Autodesk Inventor part; units mm, degrees
ref_plane "YZ Plane" through (0, 0, 0) normal (1, 0, 0) x (0, 1, 0)
ref_plane "XZ Plane" through (0, 0, 0) normal (0, 1, 0) x (-1, 0, 0)
ref_plane "XY Plane" through (0, 0, 0) normal (0, 0, 1) x (1, 0, 0)
sketch "스케치1" plane through (0, 0, 0) normal (0, 1, 0) x (-1, 0, 0)
  line L0 (24.9446, -24.9446) -> (9.1304, -34.075)
  line L1 (9.1304, -34.075) -> (-9.1304, -34.075)
  line L2 (-9.1304, -34.075) -> (-24.9446, -24.9446)
  line L3 (-24.9446, -24.9446) -> (-34.075, -9.1304)
  line L4 (-34.075, -9.1304) -> (-34.075, 9.1304)
  line L5 (-34.075, 9.1304) -> (-24.9446, 24.9446)
  line L6 (-24.9446, 24.9446) -> (-9.1304, 34.075)
  line L7 (-9.1304, 34.075) -> (9.1304, 34.075)
  line L8 (9.1304, 34.075) -> (24.9446, 24.9446)
  line L9 (24.9446, 24.9446) -> (34.075, 9.1304)
  line L10 (34.075, 9.1304) -> (34.075, -9.1304)
  line L11 (34.075, -9.1304) -> (24.9446, -24.9446)
  line L12 (9.9878, -37.275) -> (-9.9878, -37.275)
  line L13 (-9.9878, -37.275) -> (-27.2872, -27.2872)
  line L14 (-27.2872, -27.2872) -> (-37.275, -9.9878)
  line L15 (-37.275, -9.9878) -> (-37.275, 9.9878)
  line L16 (-37.275, 9.9878) -> (-27.2872, 27.2872)
  line L17 (-27.2872, 27.2872) -> (-9.9878, 37.275)
  line L18 (-9.9878, 37.275) -> (9.9878, 37.275)
  line L19 (9.9878, 37.275) -> (27.2872, 27.2872)
  line L20 (27.2872, 27.2872) -> (37.275, 9.9878)
  line L21 (37.275, 9.9878) -> (37.275, -9.9878)
  line L22 (37.275, -9.9878) -> (27.2872, -27.2872)
  line L23 (27.2872, -27.2872) -> (9.9878, -37.275)
  point P0 (0, 0)
  point P1 (0, 0)
  point P2 (0, 0)
  dimension "d0" = 70.554
  dimension "d1" = 3.2
extrude "돌출1" add sketch "스케치1" along normal blind 3.7 contours L0 L1 L2 L3 L4 L5 L6 L7 L8 L9 L10 L11 | L12 L13 L14 L15 L16 L17 L18 L19 L20 L21 L22 L23
sketch "스케치2" plane through (0, 3.7, 0) normal (0, 1, 0) x (1, 0, 0)
  line L0 (-9.5591, 35.675) -> (9.5591, 35.675)
  line L1 (9.5591, 35.675) -> (26.1159, 26.1159)
  line L2 (26.1159, 26.1159) -> (35.675, 9.5591)
  line L3 (35.675, 9.5591) -> (35.675, -9.5591)
  line L4 (35.675, -9.5591) -> (26.1159, -26.1159)
  line L5 (26.1159, -26.1159) -> (9.5591, -35.675)
  line L6 (9.5591, -35.675) -> (-9.5591, -35.675)
  line L7 (-9.5591, -35.675) -> (-26.1159, -26.1159)
  line L8 (-26.1159, -26.1159) -> (-35.675, -9.5591)
  line L9 (-35.675, -9.5591) -> (-35.675, 9.5591)
  line L10 (-35.675, 9.5591) -> (-26.1159, 26.1159)
  line L11 (-26.1159, 26.1159) -> (-9.5591, 35.675)
  line L12 (9.9878, 37.275) -> (-9.9878, 37.275)
  point P0 (0, 0)
  point P1 (0, 0)
  point P2 (0, 35.675)
  dimension "d4" = 1.6
extrude "돌출2" cut sketch "스케치2" against normal blind 1.2
sketch "스케치3" plane through (0, 2.5, 0) normal (0, 1, 0) x (1, 0, 0)
  line L0 (-9.0232, 33.675) -> (9.0232, 33.675)
  line L1 (9.0232, 33.675) -> (24.6518, 24.6518)
  line L2 (24.6518, 24.6518) -> (33.675, 9.0232)
  line L3 (33.675, 9.0232) -> (33.675, -9.0232)
  line L4 (33.675, -9.0232) -> (24.6518, -24.6518)
  line L5 (24.6518, -24.6518) -> (9.0232, -33.675)
  line L6 (9.0232, -33.675) -> (-9.0232, -33.675)
  line L7 (-9.0232, -33.675) -> (-24.6518, -24.6518)
  line L8 (-24.6518, -24.6518) -> (-33.675, -9.0232)
  line L9 (-33.675, -9.0232) -> (-33.675, 9.0232)
  line L10 (-33.675, 9.0232) -> (-24.6518, 24.6518)
  line L11 (-24.6518, 24.6518) -> (-9.0232, 33.675)
  line L12 (-9.5591, 35.675) -> (9.5591, 35.675)
  point P0 (0, 0)
  point P1 (0, 0)
  dimension "d7" = 2
extrude "돌출3" add sketch "스케치3" along normal blind 0.6
fillet "모깎기1" radius 1.2 24 edges at (-18.6375, 3.7, 32.2811) (-32.2811, 3.7, 18.6375) (-37.275, 3.7, 0) (0, 3.7, 37.275) (18.6375, 3.7, 32.2811) (32.2811, 3.7, 18.6375) (37.275, 3.7, 0) (32.2811, 3.7, -18.6375) (18.6375, 3.7, -32.2811) (0, 3.7, -37.275) (-18.6375, 3.7, -32.2811) (-32.2811, 3.7, -18.6375) (-37.275, 0, 0) (-32.2811, 0, 18.6375) (-18.6375, 0, 32.2811) (0, 0, 37.275) (18.6375, 0, 32.2811) (32.2811, 0, 18.6375) (37.275, 0, 0) (32.2811, 0, -18.6375) (18.6375, 0, -32.2811) (0, 0, -37.275) (-18.6375, 0, -32.2811) (-32.2811, 0, -18.6375)
sketch "스케치11" plane through (0, 0, 0) normal (0, -1, 0) x (1, 0, 0)
  circle A0 centre (0, 0) radius 12.7
  dimension "d48" = 25.4
extrude "돌출11" add sketch "스케치11" along normal blind 10.16
sketch "스케치12" plane through (0, -10.16, 0) normal (0, -1, 0) x (1, 0, 0)
  circle A0 centre (0, 0) radius 4.5
  line L0 (-2.5981, 4.5) -> (2.5981, 4.5)
  line L1 (2.5981, 4.5) -> (5.1962, 0)
  line L2 (5.1962, 0) -> (2.5981, -4.5)
  line L3 (2.5981, -4.5) -> (-2.5981, -4.5)
  line L4 (-2.5981, -4.5) -> (-5.1962, 0)
  line L5 (-5.1962, 0) -> (-2.5981, 4.5)
  point P0 (-3.8971, 2.25)
  point P1 (-3.8971, -2.25)
  point P2 (0, 4.5)
  point P3 (0, -4.5)
  point P4 (3.8971, -2.25)
  point P5 (3.8971, 2.25)
  dimension "d51" = 9
extrude "돌출12" cut sketch "스케치12" against normal blind 12
sketch "스케치13" plane through (0, 0, 0) normal (0, -1, 0) x (1, 0, 0)
  circle A0 centre (0, -21) radius 7.5
  circle A1 centre (18.1865, -10.5) radius 7.5
  circle A2 centre (18.1865, 10.5) radius 7.5
  circle A3 centre (0, 21) radius 7.5
  circle A4 centre (-18.1865, 10.5) radius 7.5
  circle A5 centre (-18.1865, -10.5) radius 7.5
  point P0 (0, 0)
  dimension "d56" = 15
  dimension "d57" = 21
  dimension "d60" = 360
extrude "돌출13" cut sketch "스케치13" against normal up to surface (3.1 mm away)
sketch "스케치16" plane through (0, 1.84, 0) normal (0, -1, 0) x (1, 0, 0)
  line L0 (-2.5981, 4.5) -> (2.5981, 4.5)
  line L1 (-5.1962, 0) -> (-2.5981, 4.5)
  line L2 (-2.5981, -4.5) -> (-5.1962, 0)
  line L3 (2.5981, -4.5) -> (-2.5981, -4.5)
  line L4 (5.1962, 0) -> (2.5981, -4.5)
  line L5 (2.5981, 4.5) -> (5.1962, 0)
  line L6 (-2.0207, 3.5) -> (2.0207, 3.5)
  line L7 (2.0207, 3.5) -> (4.0415, 0)
  line L8 (4.0415, 0) -> (2.0207, -3.5)
  line L9 (2.0207, -3.5) -> (-2.0207, -3.5)
  line L10 (-2.0207, -3.5) -> (-4.0415, 0)
  line L11 (-4.0415, 0) -> (-2.0207, 3.5)
  point P0 (0, 0)
  point P1 (0, 0)
  dimension "d82" = 1
extrude "돌출14" add sketch "스케치16" along normal blind 8.5
fillet "모깎기2" radius 0.5 6 edges at (0, -10.16, 4.5) (3.8971, -10.16, 2.25) (3.8971, -10.16, -2.25) (0, -10.16, -4.5) (-3.8971, -10.16, 2.25) (-3.8971, -10.16, -2.25)
equation "\"d71\" = 55deg"
properties part number "OV-PAM_n_12_bottom"
Here's how the part is built. I have some questions about the finished solid (model axes, mm). A direction names the side the tool comes from. Give positions to 0.01 mm unless a question says otherwise; leave off trailing zeros. Write each loop counter-clockwise with the first axis right and the second up, starting at its lowest first coordinate (ties: lowest second). Pieces come first, ordered by that corner, then holes. Notation, with made-up numbers: (34, 86.5) -> (40, 86.5) arc R19 cw to (40, 91.5) -> close; hole circle Ø4 at (-1.75, 54.5). An arc over 180 degrees is marked (long way). Write each question's results on one line, items separated by ' | '.
Item 1: If I drill on L1, parallel to Z at x = 6.5, y = 1; L2, parallel to Y at x = -31, z = -15; L3, parallel to Y at x = 20.5, z = -18.5, over which ranges is the centre line in solid material (lowest first)?
Output:
L1: z = -37.26 to -24.74, -17.26 to 17.26, 24.74 to 37.26 | L2: y = 0 to 2.5 | L3: y = 0 to 3.1
Item 2: For pin 1 Ø13.5 at (x, z) = (18.19, 10.5) entering from -Y; pin 2 Ø2 at (x, z) = (-16, 1) entering from +Y; pin 3 Ø3.5 at (x, y) = (0.5, -8.5) entering from +Z; pin 4 Ø6 at (y, z) = (-0.5, 21) entering from -X (3 decimals), each with a flat end and sliding along its axis, tell me the tip position at first contact or that it passes through.
Output:
pin 1: passes through | pin 2: stops at y = 3.1 | pin 3: stops at z = 12.7 | pin 4: stops at x = -32.405
Item 3: On a 3-axis mill with a long thin cutter (end or side, diameter ignored), from which of +Z, -Z, +X, -X, +Y, -Y can I reach the whole of each face in a straight line? I mean faces 4 (the face through (-32.039, 0.342, 18.336)), 5 (the face through (16.728, 2.796, -29.227)), 6 (the face through (0, -2, 3.5)). Say none if no direction works.
Output:
face 4: +Z, -X, -Y | face 5: +Y | face 6: -Y
Item 4: Suppose I cut it at B-B on z = -6. Write out the boundary of the cut face in (x, y) (1 decimal).
Output:
outline: (-37.3, 1.2) arc R1.2 ccw to (-36.1, 0) -> (-24.2, 0) -> (-24.2, 3.1) -> (-33.7, 3.1) -> (-33.7, 2.5) -> (-35.7, 2.5) -> (-35.7, 3.7) -> (-36.1, 3.7) arc R1.2 ccw to (-37.3, 2.5) -> close; (-12.2, 0) -> (-11.2, 0) -> (-11.2, -10.2) -> (11.2, -10.2) -> (11.2, 0) -> (12.2, 0) -> (12.2, 3.1) -> (-12.2, 3.1) -> close; (24.2, 0) -> (36.1, 0) arc R1.2 ccw to (37.3, 1.2) -> (37.3, 2.5) arc R1.2 ccw to (36.1, 3.7) -> (35.7, 3.7) -> (35.7, 2.5) -> (33.7, 2.5) -> (33.7, 3.1) -> (24.2, 3.1) -> close
Item 5: We'd pull the mould along X, two halves only. Please class faces 1 (the face through (18.52, 1.84, -32.35)), 2 (the face through (18, 3.1, 30.8)), 3 (the face through (-18.35, 3.34, -32.05)): pulls with the +X half, pulls with the -X half, needs draft (parallel to the pull), parting line crosses it, or undercut.
Output:
face 1: pulls with the +X half | face 2: undercut | face 3: pulls with the -X half
Item 6: Suppose I cut it at C-C on x = 0. Give the number of separate pieces and of enclosed holes in the cut face, plus the area to 3 significant figures.
Output:
separate pieces: 3 | enclosed holes: 0 | area: 303 mm^2
Item 7: Suppose I cut it at A-A on y = -8.25. Write out the boundary of the cut face in (x, z), plus the area to 3 significant figures.
Output:
outline: circle Ø25.4 at (0, 0); hole (-5.2, 0) -> (-2.6, -4.5) -> (2.6, -4.5) -> (5.2, 0) -> (2.6, 4.5) -> (-2.6, 4.5) -> close | area: 437 mm^2
